Here's how the part is built. I have some questions about the finished solid (model axes, mm). A direction names the side the tool comes from. Give positions to 0.01 mm unless a question says otherwise; leave off trailing zeros. Loops run counter-clockwise (first coordinate to the right, second up) from the corner with the lowest first, then second, coordinate; pieces in that order, holes last. Notation, with made-up numbers: (-31, 23) - (27, 23) arc R17 ccw to (27, 32) - close; hole circle Ø6 at (61.5, 75.5). An arc over 180 degrees is marked (long way). Put each result on its own line as item: value. Start each with the question number.
from build123d import *

# Parameters (mm, degrees)
SKETCH_2_R          = 29.5
EXTRUDE_1_DEPTH     = 2
SKETCH_3_R          = 25
EXTRUDE_2_DEPTH     = 10
SKETCH_7_R          = 1.4
CUT_EXTRUDE_3_DEPTH = 12
CUT_EXTRUDE_4_REACH = 45.411
SKETCH_9_R          = 6.5
EXTRUDE_START       = -5.9
SKETCH_10_R         = 6.5
SKETCH_10_R_2       = 5.5
EXTRUDE_4_DEPTH     = 5.9


with BuildPart() as part:
    # 草图2 → 凸台-拉伸1 (new body)
    with BuildSketch(Plane.XY):
        Circle(SKETCH_2_R)
    extrude(amount=EXTRUDE_1_DEPTH)

    # 草图3 → 凸台-拉伸2 (add)
    with BuildSketch(Plane.XY.offset(2)):
        Circle(SKETCH_3_R)
    extrude(amount=EXTRUDE_2_DEPTH)

    # 草图7 → 切除-拉伸3 (cut)
    with BuildSketch(Plane.XY.offset(12)):
        with Locations((12.990381057, 7.5)):
            Circle(SKETCH_7_R)
        with Locations((12.990381057, -7.5)):
            Circle(SKETCH_7_R)
        with Locations((0, -15)):
            Circle(SKETCH_7_R)
        with Locations((-12.990381057, -7.5)):
            Circle(SKETCH_7_R)
        with Locations((-12.990381057, 7.5)):
            Circle(SKETCH_7_R)
        with Locations((0, 15)):
            Circle(SKETCH_7_R)
    extrude(amount=-CUT_EXTRUDE_3_DEPTH, mode=Mode.SUBTRACT)

    # 草图9 → 切除-拉伸4 (cut, up to next)
    with BuildSketch(Plane(origin=(0, 0, 0), x_dir=(-1, 0, 0), z_dir=(0, 0, -1)), mode=Mode.PRIVATE) as cut_extrude_4_sk1:
        Circle(SKETCH_9_R)
    cut_extrude_4_tool1 = extrude(cut_extrude_4_sk1.sketch, amount=-CUT_EXTRUDE_4_REACH, mode=Mode.PRIVATE) & part.part
    add(cut_extrude_4_tool1.solids().sort_by_distance((0, 0, 0))[0], mode=Mode.SUBTRACT)

    # 草图10 → 凸台-拉伸4 (add)
    with BuildSketch(Plane.XY.offset(12).offset(EXTRUDE_START)):
        with Locations(Location((0, 0, 0), (0, 0, 180))):
            Circle(SKETCH_10_R)
        Circle(SKETCH_10_R_2, mode=Mode.SUBTRACT)
    extrude(amount=EXTRUDE_4_DEPTH)


solid = part.part
1) Suppose I cut it at C-C on x = 0. Please give me the cut outline in (y, z), plus the area to 3 significant figures.
2) Suppose I cut it at D-D on y = 7.5. Please give me the cut outline in (x, z).
3) I need wall thicknesses on line 1 (Y direction, x = 0, z = 7.25); line 2 (Y direction, x = 0, z = 4); line 3 (Z direction, x = -27, y = 6). Which ranges of each line are inside material? Lowest first, please.
4) Suppose I cut it at A-A on y = 0. Please give me the cut outline in (x, z), plus the area to 3 significant figures.
5) I'm going to push flat-ended pins straight in: P1, Ø2.5, axis at x = 0, y = -15, coming from the +Z side; P2, Ø2, axis at x = 16.5, z = 5, coming from the -Y side; P3, Ø1, axis at x = 16, y = 1.5, coming from the -Z side; P4, Ø4, axis at x = 1, z = 3, coming from the +Y side. Where does each tip first touch, or does it pass through?
6) Suppose I cut it at B-B on z = 8.75. Please give me the cut outline in (x, y), plus the area to 3 significant figures.
7) Thinking about a two-plate mould opening in X: for faces 4 (the cylindrical face through (-13.294, -8.867, 6.084)), 5 (the flat face through (-22, 13, 2)), 6 (the cylindrical face through (28.14, 8.86, 0.99)), which applies, pulls with the +X half, pulls with the -X half, needs draft (parallel to the pull), parting line crosses it, or undercut?
8) Which directions (+Z, -Z, +X, -X, +Y, -Y) give clear straight access to the entire face, cutting with the end or side of a thin tool? Please do faces 1 (the cylindrical face through (-1.19, -5.37, 9.01)), 2 (the cylindrical face through (23.846, 7.509, 6.93)), 3 (the flat face through (5, -3, 6.1)).
Ans:
1. outline: (-29.5, 0) - (-16.4, 0) - (-16.4, 12) - (-25, 12) - (-25, 2) - (-29.5, 2) - close; (-13.6, 0) - (-6.5, 0) - (-6.5, 6.1) - (-5.5, 6.1) - (-5.5, 12) - (-13.6, 12) - close; (5.5, 6.1) - (6.5, 6.1) - (6.5, 0) - (13.6, 0) - (13.6, 12) - (5.5, 12) - close; (16.4, 0) - (29.5, 0) - (29.5, 2) - (25, 2) - (25, 12) - (16.4, 12) - close
1. area: 407 mm²
2. outline: (-28.53, 0) - (-14.39, 0) - (-14.39, 12) - (-23.85, 12) - (-23.85, 2) - (-28.53, 2) - close; (-11.59, 0) - (11.59, 0) - (11.59, 12) - (-11.59, 12) - close; (14.39, 0) - (28.53, 0) - (28.53, 2) - (23.85, 2) - (23.85, 12) - (14.39, 12) - close
3. line 1: y = -25 to -16.4, -13.6 to -5.5, 5.5 to 13.6, 16.4 to 25
3. line 2: y = -25 to -16.4, -13.6 to -6.5, 6.5 to 13.6, 16.4 to 25
3. line 3: z = 0 to 2
4. outline: (-29.5, 0) - (-6.5, 0) - (-6.5, 6.1) - (-5.5, 6.1) - (-5.5, 12) - (-25, 12) - (-25, 2) - (-29.5, 2) - close; (5.5, 6.1) - (6.5, 6.1) - (6.5, 0) - (29.5, 0) - (29.5, 2) - (25, 2) - (25, 12) - (5.5, 12) - close
4. area: 474 mm²
5. P1: passes through
5. P2: stops at y = -19.62
5. P3: stops at z = 0
5. P4: stops at y = 29.5
6. outline: circle Ø50 at (0, 0); hole circle Ø2.8 at (-12.99, -7.5); hole circle Ø2.8 at (-12.99, 7.5); hole circle Ø11 at (0, 0); hole circle Ø2.8 at (0, -15); hole circle Ø2.8 at (0, 15); hole circle Ø2.8 at (12.99, -7.5); hole circle Ø2.8 at (12.99, 7.5)
6. area: 1,830 mm²
7. face 4: undercut
7. face 5: needs draft
7. face 6: parting line crosses it
8. face 1: +Z, -Z
8. face 2: +Z
8. face 3: -Z
